```python
from build123d import *

# Parameters (mm, degrees)
BOSS_EXTRU_1_DEPTH = 10
SKETCH1_R          = 3.95
CUT_EXTRUDE1_DEPTH = 8


with BuildPart() as part:
    # Esquisse1 → Boss.-Extru.1 (new body)
    with BuildSketch(Plane.XY):
        with BuildLine():
            Line((10.495334687, 9.6), (60.495334687, 5.135702408))
            ThreePointArc((60.495334687, 5.135702408), (65.192921242, 0), (60.495334687, -5.135702408))
            Line((60.495334687, -5.135702408), (10.495334687, -9.6))
            ThreePointArc((10.495334687, -9.6), (0, 0), (10.495334687, 9.6))
        make_face()
    extrude(amount=BOSS_EXTRU_1_DEPTH)

    # Sketch1 → Cut-Extrude1 (cut)
    with BuildSketch(Plane(origin=(0, 0, 0), x_dir=(-1, 0, 0), z_dir=(0, 0, -1))):
        with Locations((-10.495334687, 0)):
            Circle(SKETCH1_R)
    extrude(amount=-CUT_EXTRUDE1_DEPTH, mode=Mode.SUBTRACT)


solid = part.part
```
Work out the finished part from the listing and answer in its coordinate system (mm). Give positions to 0.01 mm unless a question says otherwise; leave off trailing zeros. Loops run counter-clockwise (first coordinate to the right, second up) from the corner with the lowest first, then second, coordinate; pieces in that order, holes last. Notation, with made-up numbers: (52, 47.25) -> (84, 47.25) arc R22 ccw to (84, 54.25) -> close; hole circle Ø7 at (18, -18.75). An arc over 180 degrees is marked (long way). Use CSV: the item, a comma, the result in double quotes.
1. The part is cut by section A-A (z = 2.5). Write down the section's boundary in (x, y).
Found:
outline,"(10.5, -9.6) -> (60.5, -5.14) arc R5.16 ccw to (60.5, 5.14) -> (10.5, 9.6) arc R9.64 ccw (long way) to start; hole circle Ø7.9 at (10.5, 0)"
2. The part is cut by section B-B (y = 0). Write down the section's boundary in (x, z), then the cut area to 3 significant figures.
Found:
outline,"(0, 0) -> (6.55, 0) -> (6.55, 8) -> (14.45, 8) -> (14.45, 0) -> (65.19, 0) -> (65.19, 10) -> (0, 10) -> close"
area,"589 mm^2"
3. Flat-ended cylindrical pins translate along their axes: pin 1 Ø8 at (x, y) = (18.5, -7.5) entering from -Z; pin 2 Ø2 at (y, z) = (-6.5, 3.5) entering from -X; pin 3 Ø3 at (x, z) = (33, 8.5) entering from +Y; pin 4 Ø6 at (x, z) = (13.5, 2) entering from -Y. Find the tip coordinate at first contact, or state that the pin passes through.
Found:
pin 1,"z = 0"
pin 2,"x = 1.72"
pin 3,"y = 7.72"
pin 4,"y = -9.6"
4. The mould has two halves that part along Y. Classify faces 1 (the flat face through (35.15, 7.4, 4.93)), 2 (the cylindrical face through (65.19, 0.11, 4.93)), 3 (the cylindrical face through (13.407, 2.67, 3.944)), 4 (the flat face through (11, 0, 8)): +Y half, -Y half, draft (parallel to the pull), parting line (faces both ways), or undercut.
Found:
face 1,"+Y half"
face 2,"parting line"
face 3,"undercut"
face 4,"undercut"
5. Straight lines are drawn through the part: line 1 (Y direction, x = 7.5, z = 1.5); line 2 (Y direction, x = 13, z = 0.75); line 3 (X direction, y = -2.5, z = 6). For each, find the intervals that lie inside material, in ascending order.
Found:
line 1,"-9.4 to -2.57, 2.57 to 9.4"
line 2,"-9.38 to -3.05, 3.05 to 9.38"
line 3,"0.33 to 7.44, 13.55 to 64.55"
6. The part is cut by section C-C (x = 29). Write down the section's boundary in (y, z).
Found:
outline,"(-7.95, 0) -> (7.95, 0) -> (7.95, 10) -> (-7.95, 10) -> close"
7. The part is cut by section D-D (y = 7.5). Write down the section's boundary in (x, z), then the cut area to 3 significant figures.
Found:
outline,"(3.58, 0) -> (34.02, 0) -> (34.02, 10) -> (3.58, 10) -> close"
area,"304 mm^2"
